```python
from build123d import *


with BuildPart() as part:
    # Sketch1 → Revolve1 (revolve)
    with BuildSketch(Plane(origin=(0, 0, 0), x_dir=(0, 0, -1), z_dir=(1, 0, 0)), mode=Mode.PRIVATE) as revolve1_sk:
        Polygon((0, 0), (0, 3.175), (2.54, 3.175), (8.89, 4.572), (8.89, 3.81), (15.24, 3.81), (15.24, 6.35), (20.32, 6.35), (20.8788, 3.81), (27.2288, 3.81), (27.2288, 4.572), (33.5788, 3.175), (36.1188, 3.175), (36.1188, 0), align=None)
    revolve(revolve1_sk.sketch.rotate(Axis((0, 0, -36.1188), (0, 0, 1)), 90), axis=Axis((0, 0, -36.1188), (0, 0, 1)))


solid = part.part
```
Can you work these out from the model? Positions are in its coordinate system, mm. A direction names the side the tool comes from. Coordinates: 2 decimals unless noted, no trailing zeros. Loops run counter-clockwise (first coordinate to the right, second up) from the corner with the lowest first, then second, coordinate; pieces in that order, holes last. Notation, with made-up numbers: M 55,39.5 L 108,39.5 A24 ccw 108,52.5 Z; hole C 17.25,20 d6. An arc over 180 degrees is marked long. Put each result on its own line as item: value. Start each with the question number.
(1) We'd pull the mould along Z, two halves only. Please class faces 1 (the face through (0, 0, 0)), 2 (the face through (0.496, -3.778, -24.098)), 3 (the face through (2.52, 1.93, -34.87)), 4 (the face through (0, 0, -36.119)): +Z half, -Z half, draft (parallel to the pull), parting line (faces both ways), or undercut.
(2) I need wall thicknesses on probe 1 along Y at (x, z) = (0.25, -31.5); probe 2 along Z at (x, y) = (5.5, 2); probe 3 along Z at (x, y) = (-4, -2.75). Which ranges of each line are inside material? Lowest first, please.
(3) Which directions (+Z, -Z, +X, -X, +Y, -Y) give clear straight access to the entire face, cutting with the end or side of a thin tool? Please do faces 5 (the face through (5.04, 3.86, -17.82)), 6 (the face through (2.52, 1.93, -1.29)), 7 (the face through (1, -4, -8.89)).
(4) Will these pins go through, and if not, where does the flat tip stop? pin 1 Ø1.5 at (y, z) = (2, -27.5) entering from +X; pin 2 Ø3 at (y, z) = (-2.5, -9) entering from +X; pin 3 Ø2 at (x, z) = (-1.5, -31.5) entering from +Y.
(5) Imagine slicing it at A-A on y = 0. List the corners of the cut face in (x, z) for me (3 decimals).
(6) Imagine slicing it at C-C on z = -17. List the corners of the cut face in (x, y) for me, and give its area (3 significant figures).
(7) Imagine slicing it at D-D on z = -13. List the corners of the cut face in (x, y) for me, and give its area (3 significant figures).
Worked answers:
1. face 1: +Z half
1. face 2: undercut
1. face 3: draft
1. face 4: -Z half
2. probe 1: y = -3.62 to 3.62
2. probe 2: z = -20.43 to -15.24
2. probe 3: z = -20.65 to -15.24
3. face 5: +Z, -Z
3. face 6: +Z
3. face 7: none
4. pin 1: stops at x = 4.38
4. pin 2: stops at x = 4.46
4. pin 3: stops at y = 3.7
5. outline: M -6.35,-20.32 L -3.81,-20.879 L -3.81,-27.229 L -4.572,-27.229 L -3.175,-33.579 L -3.175,-36.119 L 3.175,-36.119 L 3.175,-33.579 L 4.572,-27.229 L 3.81,-27.229 L 3.81,-20.879 L 6.35,-20.32 L 6.35,-15.24 L 3.81,-15.24 L 3.81,-8.89 L 4.572,-8.89 L 3.175,-2.54 L 3.175,0 L -3.175,0 L -3.175,-2.54 L -4.572,-8.89 L -3.81,-8.89 L -3.81,-15.24 L -6.35,-15.24 Z
6. outline: C 0,0 d12.7
6. area: 127 mm2
7. outline: C 0,0 d7.62
7. area: 45.6 mm2
